Study the drawing (mm; zero at the part's minimum x, y, z) and answer. A direction names the side the tool comes from. Coordinates: 2 decimals unless noted, no trailing zeros. Order: outer loops, then holes, each group sorted by start corner. A loop starts at its lowest first (then second) coordinate and runs counter-clockwise, first axis right, second up.
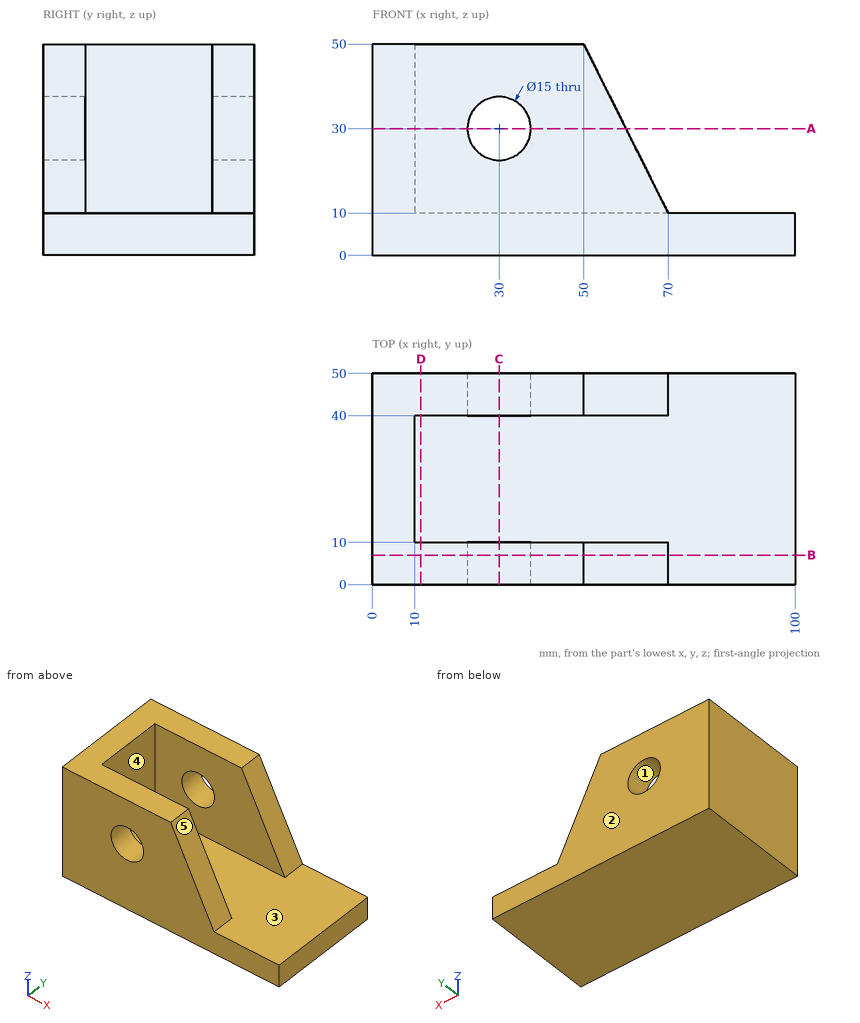
(1) Find section B-B (y = 7). Write down the section's boundary in (x, z).
(2) Consider line 1 (Z direction, x = 30, y = 47); line 2 (Y direction, x = 45.5, z = 39); line 3 (X direction, y = 21.5, z = 29). Determine where each line is inside the solid, lowest interval first.
(3) Each of these flat-tipped pins is pushed along its axis until it touches: pin 1 Ø5 at (x, z) = (68.5, 23.5) entering from +Y; pin 2 Ø3 at (x, y) = (88, 42.5) entering from +Z. Where does it stop, or does it pass through?
(4) Find section A-A (z = 30). Write down the section's boundary in (x, y), and give its area (3 significant figures).
(5) The mould has two halves that part along Z. Classify the marked faces 1, 2 and 3: released by +Z, released by -Z, zero draft, split by the parting line, or undercut.
(6) For the marked faces 4 and 5, determine the directions among +Z, -Z, +X, -X, +Y, -Y from which every point of the face is accessible in a straight line to the end or side of a thin tool.
(7) Find section C-C (x = 30). Write down the section's boundary in (y, z).
(8) Find section D-D (x = 11.5). Write down the section's boundary in (y, z), and give its area (3 significant figures).
Findings below:
1. outline: (0, 0) - (100, 0) - (100, 10) - (70, 10) - (50, 50) - (0, 50) - close; hole circle Ø15 at (30, 30)
2. line 1: z = 0 to 22.5, 37.5 to 50
2. line 2: y = 0 to 10, 40 to 50
2. line 3: x = 0 to 10
3. pin 1: passes through
3. pin 2: stops at z = 10
4. outline: (0, 0) - (22.5, 0) - (22.5, 10) - (10, 10) - (10, 40) - (22.5, 40) - (22.5, 50) - (0, 50) - close; (37.5, 0) - (60, 0) - (60, 10) - (37.5, 10) - close; (37.5, 40) - (60, 40) - (60, 50) - (37.5, 50) - close
4. area: 1,200 mm2
5. face 1: undercut
5. face 2: zero draft
5. face 3: released by +Z
6. face 4: +Z, +X
6. face 5: +Z, +X, +Y, -Y
7. outline: (0, 0) - (50, 0) - (50, 22.5) - (40, 22.5) - (40, 10) - (10, 10) - (10, 22.5) - (0, 22.5) - close; (0, 37.5) - (10, 37.5) - (10, 50) - (0, 50) - close; (40, 37.5) - (50, 37.5) - (50, 50) - (40, 50) - close
8. outline: (0, 0) - (50, 0) - (50, 50) - (40, 50) - (40, 10) - (10, 10) - (10, 50) - (0, 50) - close
8. area: 1,300 mm2
